Input: part model. Units: mm. Frame: model coordinates. Face numbers are marked on the shaded views. Coordinates: 2 decimals unless noted, no trailing zeros. Order: outer loops, then holes, each group sorted by start corner. A loop starts at its lowest first (then second) coordinate and runs counter-clockwise, first axis right, second up. Notation, with made-up numbers: (-8.75, 19.5) -> (17.25, 19.5) arc R15 ccw to (17.25, 23.5) -> close; hole circle Ø6 at (-22.5, 47.25). An arc over 180 degrees is marked (long way). Write each question's results on one line, items separated by ' | '.
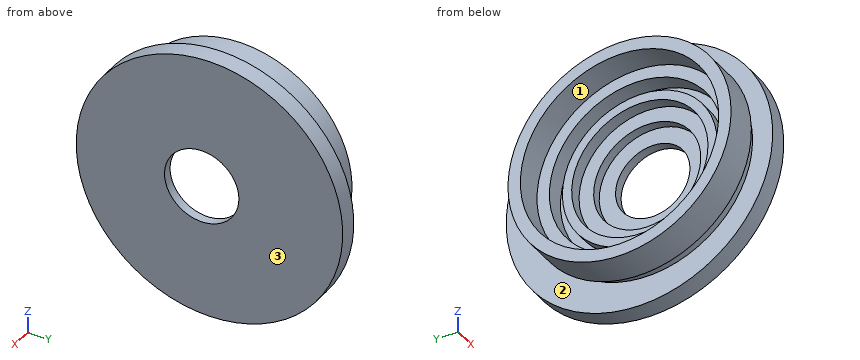
```python
from build123d import *

# Parameters (mm, degrees)
ESQUISSE2_R        = 43
ESQUISSE2_R_2      = 17.284931715
BOSS_EXTRU_1_DEPTH = 6


with BuildPart() as part:
    # Esquisse1 → Base-R_volution (revolve)
    with BuildSketch(Plane.XY, mode=Mode.PRIVATE) as base_r_volution_sk:
        Polygon((0, 12), (0, 34), (-10, 34), (-10, 36), (-21, 36), (-21, 32), (-12, 32), (-12, 28), (-4, 28), (-4, 25), (-10, 25), (-10, 22), (-4, 22), (-4, 18), (-3, 18), (-3, 12), align=None)
    revolve(base_r_volution_sk.sketch.rotate(Axis((-25.921870853, 0, 0), (1, 0, 0)), 90), axis=Axis((-25.921870853, 0, 0), (1, 0, 0)))

    # Esquisse2 → Boss.-Extru.1 (add)
    with BuildSketch(Plane(origin=(0, 0, 0), x_dir=(0, 0, -1), z_dir=(1, 0, 0))):
        with Locations((0, 2.5)):
            Circle(ESQUISSE2_R)
        Circle(ESQUISSE2_R_2, mode=Mode.SUBTRACT)
    extrude(amount=-BOSS_EXTRU_1_DEPTH)


solid = part.part
```
(1) Cut plane C-C, the plane z = -33. Return loops of the section in (x, y).
Return value:
outline: (-21, -14.39) -> (-10, -14.39) -> (-10, -8.19) -> (-6, -8.19) -> (-6, -25.07) -> (0, -25.07) -> (0, 30.07) -> (-6, 30.07) -> (-6, 8.19) -> (-10, 8.19) -> (-10, 14.39) -> (-21, 14.39) -> close
(2) Cut plane A-A, the plane x = -7.25. Return loops of the section in (y, z), plus the area to 3 significant figures.
Return value:
outline: circle Ø68 at (0, 0); circle Ø50 at (0, 0); hole circle Ø56 at (0, 0); hole circle Ø44 at (0, 0) | area: 1,610 mm2
(3) Cut plane B-B, the plane x = -13.25. Return loops of the section in (y, z).
Return value:
outline: circle Ø72 at (0, 0); hole circle Ø64 at (0, 0)
(4) Line query: line 1 along Y through (x, z) = (-8.85, 0); line 2 along Y through (x, z) = (-5.25, 0); line 3 along Y through (x, z) = (-8.75, -10). Output: solid intervals per line, ascending. Write a range as from..to.
Return value:
line 1: -34..-28, -25..-22, 22..25, 28..34 | line 2: -40.5..-17.28, 17.28..45.5 | line 3: -32.5..-26.15, -22.91..-19.6, 19.6..22.91, 26.15..32.5
(5) Mould query, pull axis X, two halves, no side actions, for the marked faces 1, 2 and 3. Classes: +X half, -X half, draft (parallel to the pull), parting line (faces both ways), or undercut.
Return value:
face 1: draft | face 2: undercut | face 3: +X half
(6) Pin query (flat end, axial travel): P1, Ø1, axis at x = -5, y = -22, coming from the +Z side; P2, Ø1, axis at y = 0.5, z = 23, coming from the -X side; P3, Ø25, axis at y = 6, z = 2, coming from the -X side; P4, Ø8, axis at y = -29.5, z = -15, coming from the +X side. Return the tip coordinate at first contact, or that it passes through.
Return value:
P1: z = 35.68 | P2: x = -10 | P3: x = -6 | P4: x = 0
